Could you check a few things on this model? Use its own coordinates, in mm. A direction names the side the tool comes from. Give positions to 0.01 mm unless a question says otherwise; leave off trailing zeros. Loops run counter-clockwise (first coordinate to the right, second up) from the corner with the lowest first, then second, coordinate; pieces in that order, holes last. Notation, with made-up numbers: M -3.75,81.5 L 29.25,81.5 A24 cw 29.25,108.5 Z; hole C -39.5,63.25 d2. An arc over 180 degrees is marked long. Use CSV: the item, a comma, the result in double quotes.
```python
from build123d import *

# Parameters (mm, degrees)
SKETCH_1_R              = 45.5
EXTRUDE_1_DEPTH         = 32
SKETCH_2_R              = 32
EXTRUDE_2_DEPTH         = 18
EXTRUDE_START           = -26
EXTRUDE_3_DEPTH         = 6
SKETCH_4_R              = 5.25
CUT_EXTRUDE_1_DEPTH     = 87.38533809
EXTRUDE_4_DEPTH         = 35
SKETCH_6_R              = 41
CUT_EXTRUDE_2_DEPTH     = 26
CUT_EXTRUDE_START       = -6
SKETCH_7_R              = 41.5
CUT_EXTRUDE_3_DEPTH     = 2
CUT_EXTRUDE_4_REACH     = 102.197
CUT_EXTRUDE_START_2     = 5
SKETCH_8_R              = 27
EXTRUDE_START_2         = -5
SKETCH_9_R              = 15
EXTRUDE_5_DEPTH         = 26
CUT_EXTRUDE_5_REACH     = 97.197
SKETCH_10_R             = 9
CHAMFER_1_SIZE          = 1
CUT_EXTRUDE_START_3     = -12
SKETCH_11_R             = 13.75
CUT_EXTRUDE_6_DEPTH     = 5
HOLE_WIZARD_M27_1_D     = 24
HOLE_WIZARD_M27_1_DEPTH = 7
CUT_EXTRUDE_START_4     = -49.5
SKETCH_14_R             = 12
CUT_EXTRUDE_7_DEPTH     = 49.5
CUT_EXTRUDE_8_REACH     = 112.346
SKETCH_15_R             = 7.5
FILLET_1_R              = 2
FILLET_2_R              = 2
FILLET_3_R              = 2


with BuildPart() as part:
    # 草图1 → 凸台-拉伸1 (new body)
    with BuildSketch(Plane.XY):
        Circle(SKETCH_1_R)
    extrude(amount=-EXTRUDE_1_DEPTH)

    # 草图2 → 凸台-拉伸2 (add)
    with BuildSketch(Plane(origin=(0, 0, -32), x_dir=(-1, 0, 0), z_dir=(0, 0, -1))):
        Circle(SKETCH_2_R)
    extrude(amount=EXTRUDE_2_DEPTH)

    # 草图3 → 凸台-拉伸3 (add)
    with BuildSketch(Plane.XY.offset(EXTRUDE_START)):
        with BuildLine():
            Line((-7.794228634, -4.5), (-41.294228634, 53.523702054))
            ThreePointArc((-41.294228634, 53.523702054), (-38, 65.817930688), (-25.705771366, 62.523702054))
            Line((-25.705771366, 62.523702054), (7.794228634, 4.5))
            ThreePointArc((7.794228634, 4.5), (4.5, -7.794228634), (-7.794228634, -4.5))
        make_face()
    extrude(amount=EXTRUDE_3_DEPTH)

    # 草图4 → 切除-拉伸1 (cut, through all)
    with BuildSketch(Plane.XY.offset(-20)):
        with Locations((-33.5, 58.023702054)):
            Circle(SKETCH_4_R)
    extrude(amount=-CUT_EXTRUDE_1_DEPTH, mode=Mode.SUBTRACT)

    # 草图5 → 凸台-拉伸4 (add, symmetric)
    with BuildSketch(Plane(origin=(0, 0, 0), x_dir=(0, 0, -1), z_dir=(1, 0, 0))):
        with BuildLine():
            Line((32, -48.25), (32, -0.188756435))
            Line((32, -0.188756435), (0, -0.188756435))
            Line((0, -0.188756435), (0, -48.25))
            ThreePointArc((0, -48.25), (16, -64.25), (32, -48.25))
        make_face()
    extrude(amount=EXTRUDE_4_DEPTH, both=True)

    # 草图6 → 切除-拉伸2 (cut)
    with BuildSketch(Plane.XY):
        Circle(SKETCH_6_R)
    extrude(amount=-CUT_EXTRUDE_2_DEPTH, mode=Mode.SUBTRACT)

    # 草图7 → 切除-拉伸3 (cut)
    with BuildSketch(Plane.XY.offset(CUT_EXTRUDE_START)):
        Circle(SKETCH_7_R)
    extrude(amount=CUT_EXTRUDE_3_DEPTH, mode=Mode.SUBTRACT)

    # 草图8 → 切除-拉伸4 (cut, up to next)
    with BuildSketch(Plane.XY.offset(-50).offset(CUT_EXTRUDE_START_2), mode=Mode.PRIVATE) as cut_extrude_4_sk1:
        Circle(SKETCH_8_R)
    cut_extrude_4_tool1 = extrude(cut_extrude_4_sk1.sketch, amount=CUT_EXTRUDE_4_REACH, mode=Mode.PRIVATE) & part.part
    add(cut_extrude_4_tool1.solids().sort_by_distance((0, 0, -45))[0], mode=Mode.SUBTRACT)

    # 草图9 → 凸台-拉伸5 (add)
    with BuildSketch(Plane.XY.offset(-45).offset(EXTRUDE_START_2)):
        with Locations(Location((0, 0, 0), (0, 0, 180))):
            Circle(SKETCH_9_R)
    extrude(amount=EXTRUDE_5_DEPTH)

    # 草图10 → 切除-拉伸5 (cut, up to next)
    with BuildSketch(Plane(origin=(0, 0, -50), x_dir=(-1, 0, 0), z_dir=(0, 0, -1)), mode=Mode.PRIVATE) as cut_extrude_5_sk1:
        Circle(SKETCH_10_R)
    cut_extrude_5_tool1 = extrude(cut_extrude_5_sk1.sketch, amount=-CUT_EXTRUDE_5_REACH, mode=Mode.PRIVATE) & part.part
    add(cut_extrude_5_tool1.solids().sort_by_distance((0, 0, -50))[0], mode=Mode.SUBTRACT)

    # 倒角1
    chamfer_1_edges = [part.edges().sort_by_distance(p)[0] for p in [
        (9, 0, -50),
    ]]
    chamfer(chamfer_1_edges, length=CHAMFER_1_SIZE)

    # 草图11 → 切除-拉伸6 (cut)
    with BuildSketch(Plane.ZY.offset(35).offset(CUT_EXTRUDE_START_3)):
        with Locations(Location((-16, -44.25, 0), (0, 0, 131.432457074))):
            Circle(SKETCH_11_R)
    extrude(amount=CUT_EXTRUDE_6_DEPTH, mode=Mode.SUBTRACT)

    # M27 螺纹孔1
    with Locations(Plane.ZY.offset(35)):
        with Locations((-16, -44.25)):
            Hole(HOLE_WIZARD_M27_1_D / 2, depth=HOLE_WIZARD_M27_1_DEPTH)

    # 草图14 → 切除-拉伸7 (cut)
    with BuildSketch(Plane.ZY.offset(23).offset(CUT_EXTRUDE_START_4)):
        with Locations((-16, -44.25)):
            Circle(SKETCH_14_R)
    extrude(amount=CUT_EXTRUDE_7_DEPTH, mode=Mode.SUBTRACT)

    # 草图15 → 切除-拉伸8 (cut, up to next)
    with BuildSketch(Plane.ZY.offset(-26.5), mode=Mode.PRIVATE) as cut_extrude_8_sk1:
        with Locations((-16, -44.25)):
            Circle(SKETCH_15_R)
    cut_extrude_8_tool1 = extrude(cut_extrude_8_sk1.sketch, amount=-CUT_EXTRUDE_8_REACH, mode=Mode.PRIVATE) & part.part
    add(cut_extrude_8_tool1.solids().sort_by_distance((26.5, -44.25, -16))[0], mode=Mode.SUBTRACT)

    # 圆角1
    fillet_1_edges = [part.edges().sort_by_distance(p)[0] for p in [
        (-14.506275845, 43.125606791, -23),
        (-22.75, 39.404155872, -20),
        (-30.094733113, 34.125606791, -23),
        (-22.75, 39.404155872, -26),
    ]]
    fillet(fillet_1_edges, radius=FILLET_1_R)

    # 圆角2
    fillet_2_edges = [part.edges().sort_by_distance(p)[0] for p in [
        (-15.455581516, 42.794567412, -32),
        (32.000000002, 0, -32),
    ]]
    fillet(fillet_2_edges, radius=FILLET_2_R)

    # 圆角3
    fillet_3_edges = [part.edges().sort_by_distance(p)[0] for p in [
        (-27, 0, -45),
        (15, 0, -45),
    ]]
    fillet(fillet_3_edges, radius=FILLET_3_R)


solid = part.part
```
1. I want a section at D-D, the plane x = -37. Give the number of separate pieces and of enclosed holes in the cut face, then the cut area to 3 significant figures.
Outcome:
separate pieces,"3"
enclosed holes,"0"
area,"843 mm2"
2. I want a section at B-B, the plane z = -38. List the corners of the cut face in (x, y) for me, then the cut area to 3 significant figures.
Outcome:
outline,"C 0,0 d64; C 0,0 d30; hole C 0,0 d54; hole C 0,0 d18"
area,"1,380 mm2"
3. Which directions (+Z, -Z, +X, -X, +Y, -Y) give clear straight access to the entire face, cutting with the end or side of a thin tool? Please do faces 1 (the face through (-31.45, -43.72, -4.01)), 2 (the face through (-25, -58, -16)), 3 (the face through (-5.85, -26.36, -34.62)), 4 (the face through (-29, 52, -20)), 5 (the face through (-36.02, 44.39, -23.04)).
Outcome:
face 1,"-X"
face 2,"none"
face 3,"+Z"
face 4,"+Z, -X, +Y"
face 5,"+Z, -Z, -X"
4. I want a section at A-A, the plane y = -44.25. List the corners of the cut face in (x, z) for me, then the cut area to 3 significant figures.
Outcome:
outline,"M -35,-32 L 35,-32 L 35,-23.5 L 26.5,-23.5 L 26.5,-28 L -23,-28 L -23,-29.75 L -28,-29.75 L -28,-28 L -35,-28 Z; M -35,-4 L -28,-4 L -28,-2.25 L -23,-2.25 L -23,-4 L 26.5,-4 L 26.5,-8.5 L 35,-8.5 L 35,0 L -35,0 Z"
area,"619 mm2"
5. I'm going to push flat-ended pins straight in: pin 1 Ø13.5 at (x, y) = (-35.5, 46.5) entering from -Z; pin 2 Ø6 at (x, y) = (14.5, 16.5) entering from +Z; pin 3 Ø16 at (y, z) = (-42, -23) entering from -X; pin 4 Ø8.5 at (x, y) = (-33.5, 58.02) entering from +Z. Where does each tip first touch, or does it pass through?
Outcome:
pin 1,"z = -26"
pin 2,"z = -45"
pin 3,"x = -35"
pin 4,"through"
6. If we mould it in two halves opening along X, with no side actions, what happens to faces 6 (the face through (-38.2, 65.7, -23)), 7 (the face through (26.5, -49, -22)), 8 (the face through (-28, -55, -22)), 9 (the face through (-5.402, 41.147, -5.014))? For each: +X half, -X half, draft (parallel to the pull), parting line (faces both ways), or undercut.
Outcome:
face 6,"parting line"
face 7,"-X half"
face 8,"undercut"
face 9,"undercut"
7. I want a section at C-C, the plane z = -16. List the corners of the cut face in (x, y) for me, then the cut area to 3 significant figures.
Outcome:
outline,"M -35,-64.25 L 35,-64.25 L 35,-51.75 L 26.5,-51.75 L 26.5,-56.25 L -23,-56.25 L -23,-58 L -28,-58 L -28,-56.25 L -35,-56.25 Z; M -35,-32.25 L -28,-32.25 L -28,-30.5 L -27.4,-30.5 A41 cw long 25.32,-32.25 L 26.5,-32.25 L 26.5,-36.75 L 35,-36.75 L 35,-29.07 A45.5 ccw long -35,-29.07 Z"
area,"1,570 mm2"
8. Please list where these lines run through material, in increasing order: line 1 (Y direction, x = 0, z = -39.25); line 2 (Z direction, x = 0.5, y = -30); line 3 (Z direction, x = 18.5, y = 33).
Outcome:
line 1,"-32 to -27, -15 to -9, 9 to 15, 27 to 32"
line 2,"-50 to -26"
line 3,"-32 to -26"
